Can you work these out from the model? Positions are in its coordinate system, mm. A direction names the side the tool comes from. Give positions to 0.01 mm unless a question says otherwise; leave off trailing zeros. Order: outer loops, then holes, each group sorted by start corner. A loop starts at its lowest first (then second) coordinate and runs counter-clockwise, first axis right, second up. Notation, with made-up numbers: M 53.5,78 L 66.5,78 A15 ccw 66.5,98 Z; hole C 78,31 d3. An arc over 180 degrees is marked long. Use one line per item in the form item = value. Start each with the question number.
1. I want a section at A-A, the plane x = 0. List the corners of the cut face in (y, z) for me.
2. I want a section at D-D, the plane x = 5.75. List the corners of the cut face in (y, z) for me.
3. I want a section at C-C, the plane y = 4. List the corners of the cut face in (x, z) for me.
4. We'd pull the mould along X, two halves only. Please class faces 1 (the face through (-0.91, 2.9, -2.88)), 2 (the face through (0, -5, 6)), 3 (the face through (-2.44, 0.99, -0.54)): +X half, -X half, draft (parallel to the pull), parting line (faces both ways), or undercut.
5. Will these pins go through, and if not, where does the flat tip stop? P1, Ø1.5, axis at x = -1, y = -2, coming from the -Z side; P2, Ø4.5, axis at x = 0, z = 0, coming from the +Y side; P3, Ø6, axis at y = 4, z = 4.5, coming from the -X side; P4, Ø3, axis at x = -2, z = -0.5, coming from the -Y side.
6. I need wall thicknesses on L1, parallel to X at y = 1.05, z = 0; L2, parallel to Y at x = 3.75, z = 4.5; L3, parallel to X at y = -1.5, z = -5.5. Which ranges of each line are inside material? Lowest first, please.
7. I want a section at B-B, the plane z = 0. List the corners of the cut face in (x, y) for me, and give its area (3 significant figures).
8. For faces 4 (the face through (0, -5, -6)), 5 (the face through (0, -3, -5.1)), which set-ups out of +Z, -Z, +X, -X, +Y, -Y let a thin tool reach every point of the face, with its end or its side?
```python
from build123d import *
from build123d.topology import SkipClean

# Parameters (mm, degrees)
SKETCH7_R           = 7.5
SKETCH7_R_2         = 2.5
BOSS_EXTRUDE3_DEPTH = 2
BOSS_EXTRUDE4_START = 5
BOSS_EXTRUDE4_DEPTH = 5


with BuildPart() as part:
    # Sketch7 → Boss-Extrude3 (new body)
    with BuildSketch(Plane(origin=(0, 0, 0), x_dir=(1, 0, 0), z_dir=(0, 1, 0))):
        with Locations(Location((0, 0, 0), (0, 0, 270))):
            Circle(SKETCH7_R)
        with Locations(Location((0, 0, 0), (0, 0, 270))):
            Circle(SKETCH7_R_2, mode=Mode.SUBTRACT)
    extrude(amount=BOSS_EXTRUDE3_DEPTH)

    # Sketch8 → Boss-Extrude4 (add)
    with SkipClean():  # the faces are left unmerged after this step: merging them gives an invalid solid
        with BuildSketch(Plane.XZ.offset(BOSS_EXTRUDE4_START)):
            with BuildLine():
                ThreePointArc((5.499090834, 5.1), (0, 7.5), (-5.499090834, 5.1))
                Line((-5.499090834, 5.1), (5.499090834, 5.1))
            make_face()
            with BuildLine():
                Line((5.499090834, -5.1), (-5.499090834, -5.1))
                ThreePointArc((-5.499090834, -5.1), (0, -7.5), (5.499090834, -5.1))
            make_face()
        extrude(amount=-BOSS_EXTRUDE4_DEPTH)

    # Sketch9 → Revolve1 (revolve)
    with SkipClean():  # the faces are left unmerged after this step: merging them gives an invalid solid
        with BuildSketch(Plane.XY, mode=Mode.PRIVATE) as revolve1_sk:
            Polygon((2.5, 2), (5.5, 7.196152423), (7.5, 7.196152423), (7.5, 2), align=None)
        revolve(revolve1_sk.sketch.rotate(Axis((0, 0, 0), (0, 1, 0)), 90), axis=Axis((0, 0, 0), (0, 1, 0)))


solid = part.part
```
Check result:
q1.outline = M -5,-7.5 L 7.2,-7.5 L 7.2,-5.5 L 2,-2.5 L 0,-2.5 L 0,-5.1 L -5,-5.1 Z; M -5,5.1 L 0,5.1 L 0,2.5 L 2,2.5 L 7.2,5.5 L 7.2,7.5 L -5,7.5 Z
q2.outline = M 0,-4.82 L 7.2,-4.82 L 7.2,4.82 L 0,4.82 Z
q3.outline = C 0,0 d15; hole C 0,0 d7.31
q4.face_1 = undercut
q4.face_2 = draft
q4.face_3 = undercut
q5.P1 = -7.5
q5.P2 = through
q5.P3 = -7.35
q5.P4 = 0
q6.L1 = -7.5 to -2.5, 2.5 to 7.5
q6.L2 = 0 to 7.2
q6.L3 = -5.1 to 5.1
q7.outline = M -7.5,0 L -2.5,0 L -2.5,2 L -5.5,7.2 L -7.5,7.2 Z; M 2.5,0 L 7.5,0 L 7.5,7.2 L 5.5,7.2 L 2.5,2 Z
q7.area = 56.4 mm2
q8.face_4 = +Z, -Z, +X, -X, -Y
q8.face_5 = +X, -X, -Y
